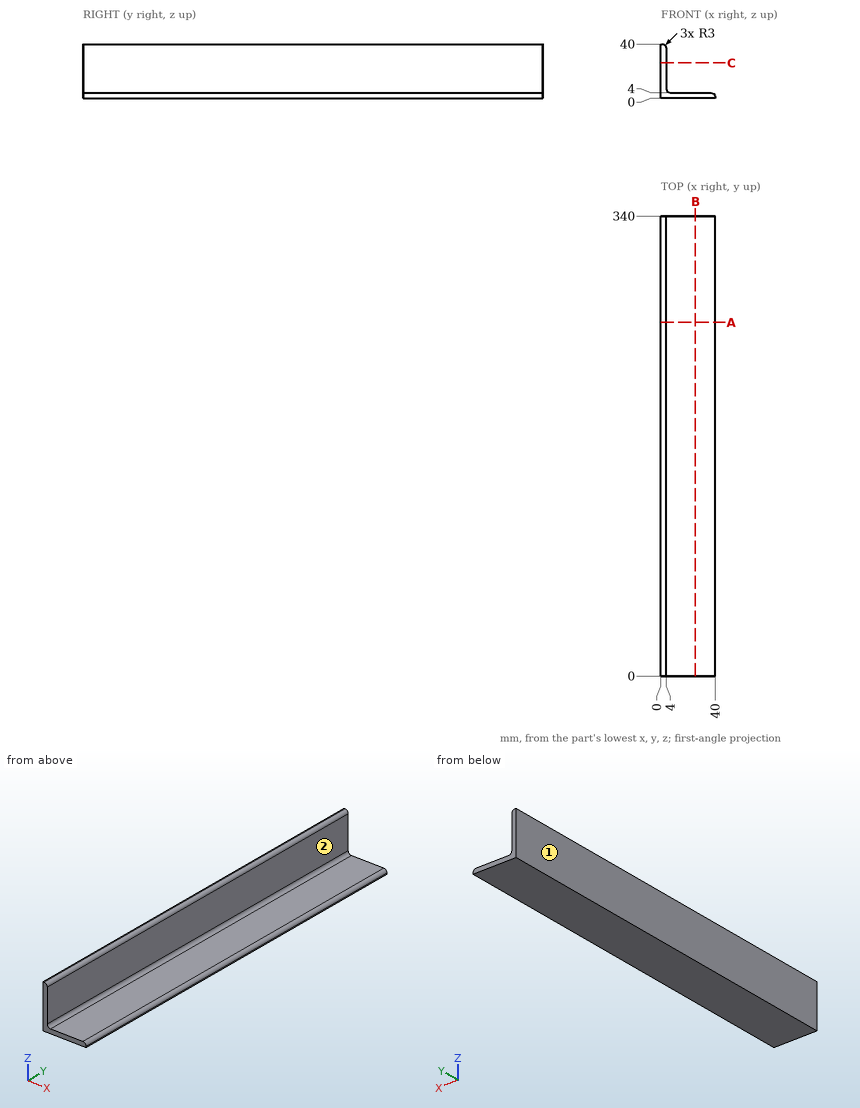
Can you work these out from the drawing? Everything is in mm from the part's minimum corner. A direction names the side the tool comes from. Coordinates: 2 decimals unless noted, no trailing zeros. Write each loop counter-clockwise with the first axis right and the second up, starting at its lowest first coordinate (ties: lowest second). Pieces come first, ordered by that corner, then holes. Notation, with made-up numbers: (83.25, 26.25) - (127.25, 26.25) arc R23 cw to (127.25, 52.25) - close; hole circle Ø2 at (28, 40). An arc over 180 degrees is marked (long way). Use a Markdown table: item, result.
Q1. Which directions (+Z, -Z, +X, -X, +Y, -Y) give clear straight access to the entire face, cutting with the end or side of a thin tool? Please do the marked faces 1 and 2.
Geometry check:
| item | result |
|---|---|
| face 1 | +Z, -Z, -X, +Y, -Y |
| face 2 | +Z, +X, +Y, -Y |
Q2. Imagine slicing it at A-A (y = 261.5). List the corners of the cut face in (x, z) for me, and give its area (3 significant figures).
Geometry check:
| item | result |
|---|---|
| outline | (0, 0) - (40, 0) - (40, 1) arc R3 ccw to (37, 4) - (7, 4) arc R3 cw to (4, 7) - (4, 37) arc R3 ccw to (1, 40) - (0, 40) - close |
| area | 302 mm2 |
Q3. I'm going to push flat-ended pins straight in: pin 1 Ø24 at (y, z) = (247, 18) entering from +X; pin 2 Ø3 at (x, y) = (17.5, 59.5) entering from +Z; pin 3 Ø6 at (y, z) = (192.5, 33) entering from +X. Where does each tip first touch, or does it pass through?
Geometry check:
| item | result |
|---|---|
| pin 1 | stops at x = 4.17 |
| pin 2 | stops at z = 4 |
| pin 3 | stops at x = 4 |
Q4. Please list where these lines run through material, in increasing order: L1, parallel to X at y = 256, z = 16; L2, parallel to X at y = 188.5, z = 38.
Geometry check:
| item | result |
|---|---|
| L1 | x = 0 to 4 |
| L2 | x = 0 to 3.83 |
Q5. Imagine slicing it at B-B (x = 25.5). List the corners of the cut face in (y, z) for me, and give its area (3 significant figures).
Geometry check:
| item | result |
|---|---|
| outline | (0, 0) - (340, 0) - (340, 4) - (0, 4) - close |
| area | 1,360 mm2 |
Q6. Imagine slicing it at C-C (z = 26). List the corners of the cut face in (x, y) for me, and give its area (3 significant figures).
Geometry check:
| item | result |
|---|---|
| outline | (0, 0) - (4, 0) - (4, 340) - (0, 340) - close |
| area | 1,360 mm2 |
